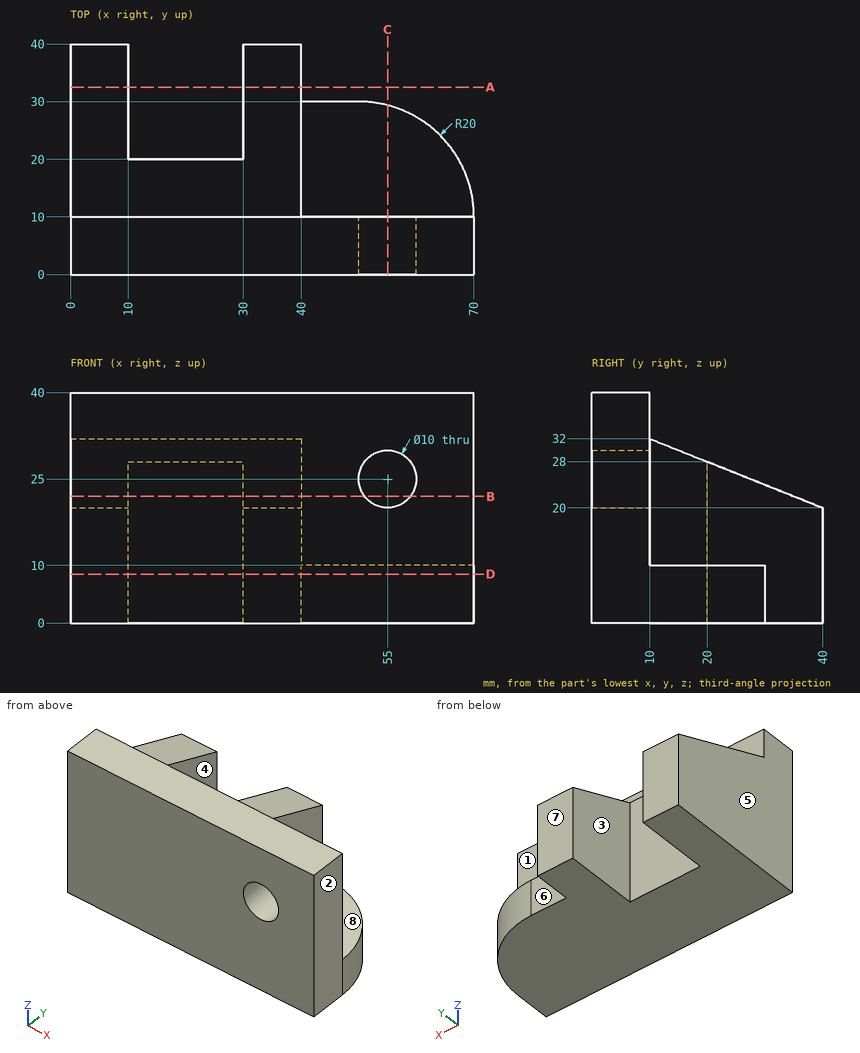
Answer from the drawing. Dimensions are ordinates in mm from the lowest x, y and z of the part. A direction names the side the tool comes from. Give positions to 0.01 mm unless a question says otherwise; leave off trailing zeros. Loops run counter-clockwise (first coordinate to the right, second up) from the corner with the lowest first, then second, coordinate; pieces in that order, holes last. Notation, with made-up numbers: (45.25, 29.5) - (77.25, 29.5) arc R34 ccw to (77.25, 60.5) - close; hole circle Ø10 at (4.5, 59.25). An arc over 180 degrees is marked (long way). Answer as a JSON object with one key per item and string values.
1. A cutting plane is placed at A-A (y = 32.5). Write down the section's boundary in (x, z), then the cut area to 3 significant figures.
Determined:
{"outline": "(0, 0) - (10, 0) - (10, 23) - (0, 23) - close; (30, 0) - (40, 0) - (40, 23) - (30, 23) - close", "area": "460 mm²"}
2. A cutting plane is placed at D-D (z = 8.5). Write down the section's boundary in (x, y).
Determined:
{"outline": "(0, 0) - (70, 0) - (70, 10) arc R20 ccw to (50, 30) - (40, 30) - (40, 40) - (30, 40) - (30, 20) - (10, 20) - (10, 40) - (0, 40) - close"}
3. A cutting plane is placed at B-B (z = 22). Write down the section's boundary in (x, y).
Determined:
{"outline": "(0, 0) - (51, 0) - (51, 10) - (40, 10) - (40, 35) - (30, 35) - (30, 20) - (10, 20) - (10, 35) - (0, 35) - close; (59, 0) - (70, 0) - (70, 10) - (59, 10) - close"}
4. For a pull along X with two mould halves and no side action, classify the marked faces 1, 2 and 3 as pulls with the +X half, pulls with the -X half, needs draft (parallel to the pull), parting line crosses it, or undercut.
Determined:
{"face 1": "needs draft", "face 2": "pulls with the +X half", "face 3": "undercut"}
5. Find the intervals of material crossed by L1, parallel to Z at x = 55, y = 6; L2, parallel to X at y = 4, z = 25; L3, parallel to X at y = 33, z = 13.5, in increasing order. Write a range as [from, to].
Determined:
{"L1": "[0, 20], [30, 40]", "L2": "[0, 50], [60, 70]", "L3": "[0, 10], [30, 40]"}
6. A cutting plane is placed at C-C (x = 55). Write down the section's boundary in (y, z), then the cut area to 3 significant figures.
Determined:
{"outline": "(0, 0) - (29.36, 0) - (29.36, 10) - (10, 10) - (10, 20) - (0, 20) - close; (0, 30) - (10, 30) - (10, 40) - (0, 40) - close", "area": "494 mm²"}
7. For the marked faces 4, 5, 6, 7 and 8, determine the directions among +Z, -Z, +X, -X, +Y, -Y from which every point of the face is accessible in a straight line to the end or side of a thin tool.
Determined:
{"face 4": "+Z, -Z, +Y", "face 5": "+Z, -Z, -X, +Y, -Y", "face 6": "+Z, -Z, +X, +Y", "face 7": "+Z, -Z, +X, -X, +Y", "face 8": "+Z, +X, +Y"}
8. Flat-ended cylindrical pins translate along their axes: pin 1 Ø3 at (x, y) = (13.5, 14.5) entering from -Z; pin 2 Ø1 at (x, z) = (18.5, 19.5) entering from +Y; pin 3 Ø16 at (y, z) = (31, 19) entering from +X; pin 4 Ø1.5 at (x, y) = (34.5, 19) entering from +Z. Find the tip coordinate at first contact, or state that the pin passes through.
Determined:
{"pin 1": "z = 0", "pin 2": "y = 20", "pin 3": "x = 40", "pin 4": "z = 28.7"}
